Part print with two shaded views. Sizes in mm from the minimum x, y, z corner. A direction names the side the tool comes from. Round coordinates to 2 decimals unless told otherwise and drop trailing zeros. Write each loop counter-clockwise with the first axis right and the second up, starting at its lowest first coordinate (ties: lowest second). Pieces come first, ordered by that corner, then holes. Notation, with made-up numbers: (87.25, -38) -> (109.25, -38) arc R13 cw to (109.25, -31) -> close; hole circle Ø6 at (87.25, -13.75). An arc over 180 degrees is marked (long way). Put each result on its own line as item: value. Start each with the question number.
1. 3-axis set-ups, long thin cutter, end or side, ignore diameter. For the marked faces 1 and 2: which of +Z, -Z, +X, -X, +Y, -Y reach the whole face in a straight line?
2. Saw through at B-B on x = 20. List the corners of the cut face in (y, z), and give its area (3 significant figures).
3. Saw through at D-D on z = 2. List the corners of the cut face in (x, y).
4. Drill centre lines: line 1 (Y direction, x = 60, z = 1.3); line 2 (Y direction, x = 20, z = 9); line 3 (Z direction, x = 22, y = 21). Where is each one in solid material? Low to high. Write a range as from..to.
5. Flat gauge pin, fed straight in: P1, Ø1.5, axis at x = 55, y = 13, coming from the +Z side. Where does the tip first touch, or does it go through?
6. Saw through at A-A on y = 10. List the corners of the cut face in (x, z).
7. Saw through at C-C on z = 5.75. List the corners of the cut face in (x, y).
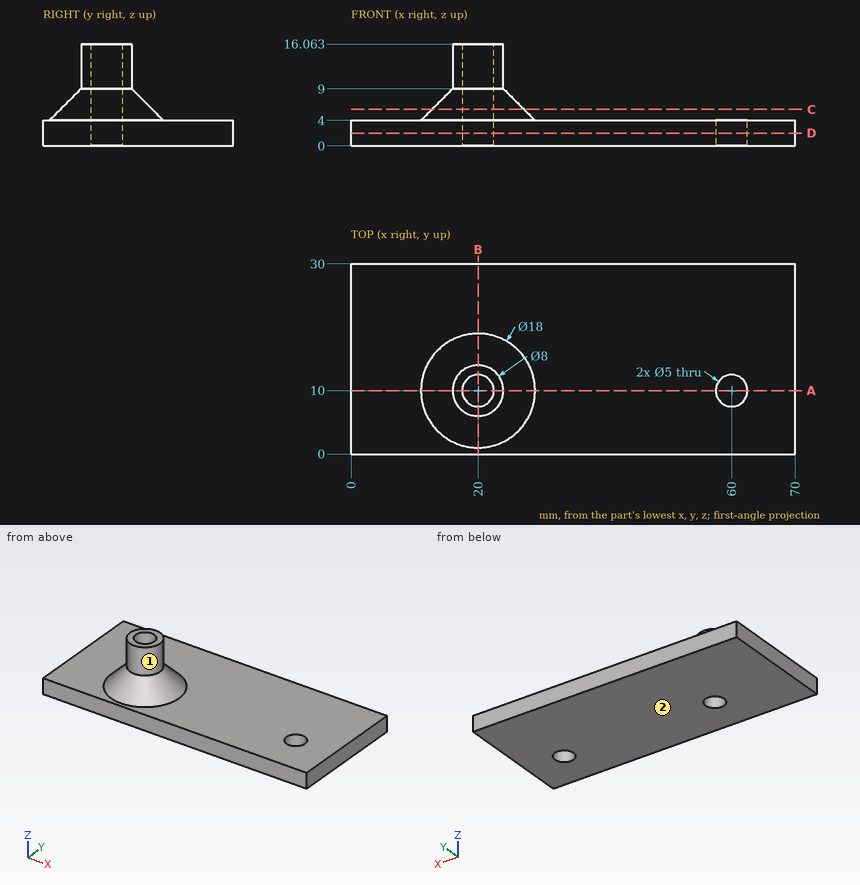
Return value:
1. face 1: +Z
1. face 2: -Z, +X, -X, +Y, -Y
2. outline: (0, 0) -> (7.5, 0) -> (7.5, 16.06) -> (6, 16.06) -> (6, 9) -> (1, 4) -> (0, 4) -> close; (12.5, 0) -> (30, 0) -> (30, 4) -> (19, 4) -> (14, 9) -> (14, 16.06) -> (12.5, 16.06) -> close
2. area: 161 mm^2
3. outline: (0, 0) -> (70, 0) -> (70, 30) -> (0, 30) -> close; hole circle Ø5 at (20, 10); hole circle Ø5 at (60, 10)
4. line 1: y = 0..7.5, 12.5..30
4. line 2: y = 6..7.5, 12.5..14
4. line 3: z = 0..4
5. P1: stops at z = 4
6. outline: (0, 0) -> (17.5, 0) -> (17.5, 16.06) -> (16, 16.06) -> (16, 9) -> (11, 4) -> (0, 4) -> close; (22.5, 0) -> (57.5, 0) -> (57.5, 4) -> (29, 4) -> (24, 9) -> (24, 16.06) -> (22.5, 16.06) -> close; (62.5, 0) -> (70, 0) -> (70, 4) -> (62.5, 4) -> close
7. outline: circle Ø14.5 at (20, 10); hole circle Ø5 at (20, 10)
